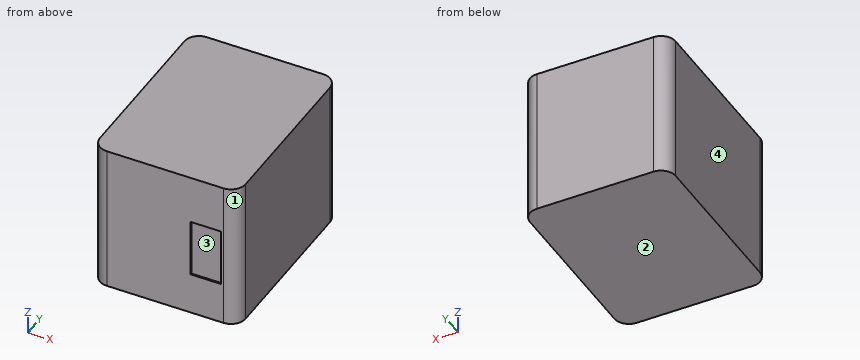
from build123d import *

# Parameters (mm, degrees)
F0_W     = 200
F0_H     = 260
F1_DEPTH = 205
F2_R     = 20
F3_W     = 42
F3_H     = 80
F4_DEPTH = 2


with BuildPart() as f1:
    # F0 (on Top) → F1 (new body)
    with BuildSketch(Plane.XY):
        with Locations((100, 130)):
            Rectangle(F0_W, F0_H)
    extrude(amount=F1_DEPTH)

    # F2
    f2_edges = [f1.edges().sort_by_distance(p)[0] for p in [
        (0, 0, 102.5),
        (0, 260, 102.5),
        (200, 260, 102.5),
        (200, 0, 102.5),
    ]]
    fillet(f2_edges, radius=F2_R)

    # F3 (on face) → F4 (cut)
    with BuildSketch(Plane.XZ):
        with Locations((156, 98)):
            Rectangle(F3_W, F3_H)
    extrude(amount=-F4_DEPTH, mode=Mode.SUBTRACT)


solid = f1.part
The model under review builds one solid part; all positions refer to its coordinate system, in mm. Face numbers are marked on the shaded views. Round coordinates to 2 decimals unless told otherwise and drop trailing zeros. Use CSV: the item, a comma, the result in double quotes.
(1) The part is to be moulded in two halves that separate along X. For the marked faces 1, 2, 3 and 4, say which applies: pulls with the +X half, pulls with the -X half, needs draft (parallel to the pull), parting line crosses it, or undercut.
Working result:
face 1,"pulls with the +X half"
face 2,"needs draft"
face 3,"undercut"
face 4,"pulls with the -X half"
(2) For line 1 (Y direction, x = 144, z = 123); line 2 (Y direction, x = 191.5, z = 97.5); line 3 (X direction, y = 247.5, z = 72.5), list the stretches that pass through material, from the lowest coordinate up.
Working result:
line 1,"y = 2 to 260"
line 2,"y = 3.64 to 256.36"
line 3,"x = 1.46 to 198.54"
(3) Clearance check with flat-ended pins moving along their axes: P1, Ø0.6, axis at y = 1.5, z = 110.5, coming from the -X side; P2, Ø10, axis at x = 160.5, y = 158, coming from the -Z side; P3, Ø0.6, axis at y = 1.5, z = 107, coming from the +X side; P4, Ø12.5, axis at x = 161.5, z = 83.5, coming from the -Y side. State where each tip first meets the part, or that it passes through.
Working result:
P1,"stops at x = 11.71"
P2,"stops at z = 0"
P3,"stops at x = 188.29"
P4,"stops at y = 2"
